Verification items for this drawing (mm, ordinates from the low corner). Give positions to 0.01 mm unless a question says otherwise; leave off trailing zeros. Write each loop counter-clockwise with the first axis right and the second up, starting at its lowest first coordinate (ties: lowest second). Pieces come first, ordered by that corner, then holes. Notation, with made-up numbers: M 22.5,-7.75 L 47.5,-7.75 A19 cw 47.5,-0.75 Z; hole C -33,76 d2. An arc over 180 degrees is marked long. Use one line per item in the form item = value. Start each with the question number.
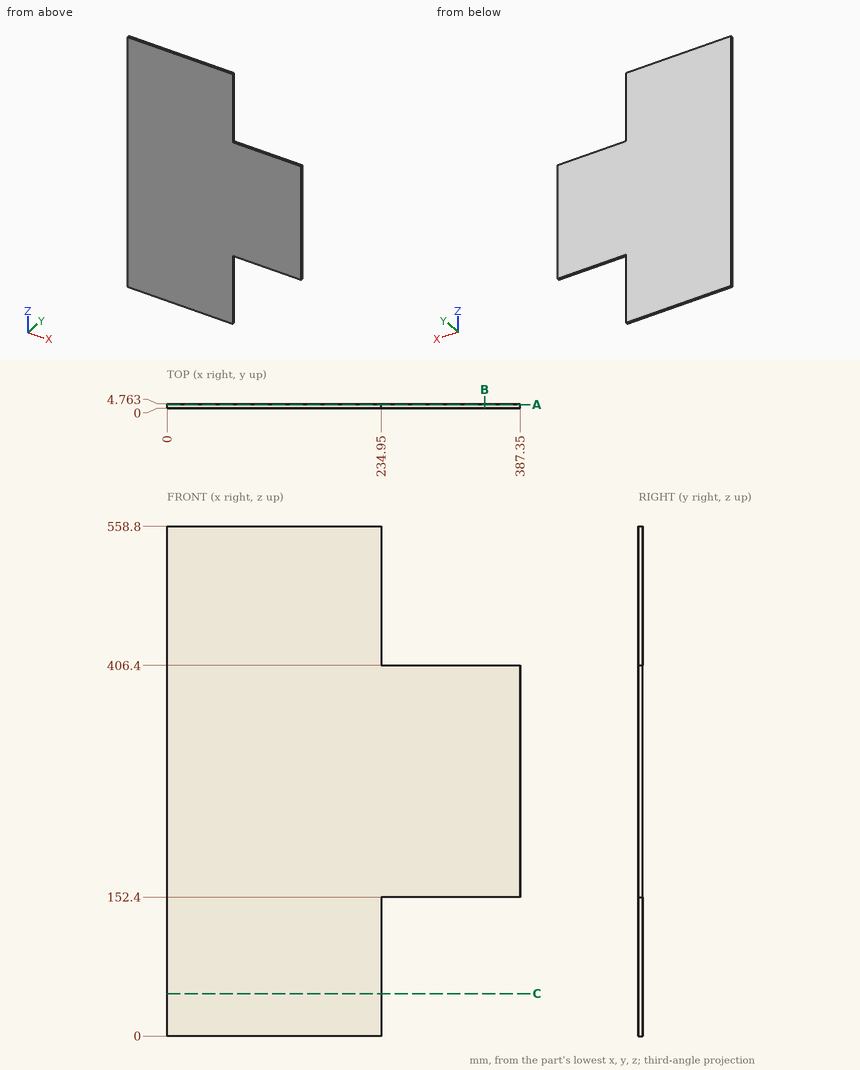
(1) Sectioned sample at C-C, the plane z = 46.5. Record the boundary of the cut face in (x, y).
(2) Thickness scan on probe 1 along X at (y, z) = (4.4, 518); probe 2 along Z at (x, y) = (261, 4.25). Record the ranges inside material, lowest first. Write a range as [from, to].
(3) Depth check by flat-ended pin: pin 1 (2.5 mm diameter, centred on x = 309.5, y = 3, fed in from +Z). Enter the tip coordinate at first touch or a pass-through.
(4) Sectioned sample at B-B, the plane x = 348. Record the boundary of the cut face in (y, z), plus the area to 3 significant figures.
(5) Sectioned sample at A-A, the plane y = 4. Record the boundary of the cut face in (x, z), plus the area to 3 significant figures.
Numbers:
q1.outline = M 0,0 L 234.95,0 L 234.95,4.76 L 0,4.76 Z
q2.probe_1 = [0, 234.95]
q2.probe_2 = [152.4, 406.4]
q3.pin_1 = 406.4
q4.outline = M 0,152.4 L 4.76,152.4 L 4.76,406.4 L 0,406.4 Z
q4.area = 1,210 mm2
q5.outline = M 0,0 L 234.95,0 L 234.95,152.4 L 387.35,152.4 L 387.35,406.4 L 234.95,406.4 L 234.95,558.8 L 0,558.8 Z
q5.area = 170,000 mm2
